Here's the drawing with two shaded views (mm, measured from the low corner). I have some questions. A direction names the side the tool comes from. Coordinates: 2 decimals unless noted, no trailing zeros. Write each loop counter-clockwise with the first axis right and the second up, starting at its lowest first coordinate (ties: lowest second). Pieces come first, ordered by that corner, then holes.
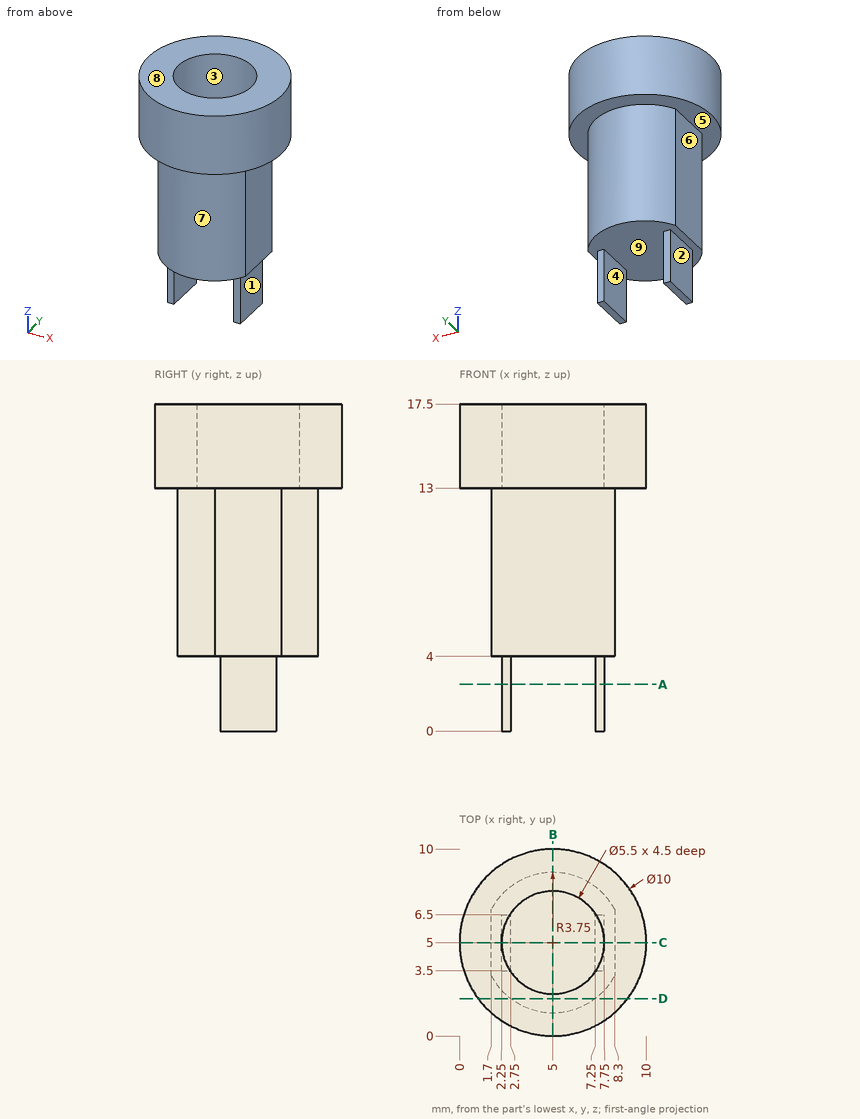
1. I want a section at D-D on y = 2. Please give me the cut outline in (x, z).
Verdict:
outline: (1, 13) - (2.75, 13) - (2.75, 4) - (7.25, 4) - (7.25, 13) - (9, 13) - (9, 17.5) - (1, 17.5) - close
2. On a 3-axis mill with a long thin cutter (end or side, diameter ignored), from which of +Z, -Z, +X, -X, +Y, -Y can I reach the whole of each face in a straight line? I mean the marked faces 1, 2, 3, 4 and 5. Say none if no direction works.
Verdict:
face 1: -Z, +X, +Y, -Y
face 2: -Z, -X, +Y, -Y
face 3: +Z
face 4: -Z, +Y, -Y
face 5: -Z
3. I want a section at B-B on x = 5. Please give me the cut outline in (y, z).
Verdict:
outline: (0, 13) - (1.25, 13) - (1.25, 4) - (8.75, 4) - (8.75, 13) - (10, 13) - (10, 17.5) - (7.75, 17.5) - (7.75, 13) - (2.25, 13) - (2.25, 17.5) - (0, 17.5) - close
4. For pin 1 (0.6 mm diameter, centred on x = 7.5, z = 2, fed in from +Y); pin 2 (1.6 mm diameter, centred on x = 5, y = 6, fed in from +Z); pin 3 (3 mm diameter, centred on x = 4.5, y = 5, fed in from -Z), each with a flat end and sliding along its axis, tell me the tip position at first contact or that it passes through.
Verdict:
pin 1: stops at y = 6.5
pin 2: stops at z = 13
pin 3: stops at z = 4
5. I want a section at A-A on z = 2.5. Please give me the cut outline in (x, y), plus the area to 3 significant figures.
Verdict:
outline: (2.25, 3.5) - (2.75, 3.5) - (2.75, 6.5) - (2.25, 6.5) - close; (7.25, 3.5) - (7.75, 3.5) - (7.75, 6.5) - (7.25, 6.5) - close
area: 3.00 mm2
6. I want a section at C-C on y = 5. Please give me the cut outline in (x, z), plus the area to 4 significant figures.
Verdict:
outline: (0, 13) - (1.7, 13) - (1.7, 4) - (2.25, 4) - (2.25, 0) - (2.75, 0) - (2.75, 4) - (7.25, 4) - (7.25, 0) - (7.75, 0) - (7.75, 4) - (8.3, 4) - (8.3, 13) - (10, 13) - (10, 17.5) - (7.75, 17.5) - (7.75, 13) - (2.25, 13) - (2.25, 17.5) - (0, 17.5) - close
area: 83.65 mm2
7. If we mould it in two halves opening along X, with no side actions, what happens to the marked faces 6, 7, 8 and 9? For each: pulls with the +X half, pulls with the -X half, needs draft (parallel to the pull), parting line crosses it, or undercut.
Verdict:
face 6: pulls with the -X half
face 7: parting line crosses it
face 8: needs draft
face 9: undercut
8. Please list where these lines run through material, in increasing order: line 1 along Y through (x, z) = (5, 14.2); line 2 along X through (y, z) = (4.75, 2); line 3 along Z through (x, y) = (4.25, 7.5).
Verdict:
line 1: y = 0 to 2.25, 7.75 to 10
line 2: x = 2.25 to 2.75, 7.25 to 7.75
line 3: z = 4 to 13
